```python
from build123d import *

# Parameters (mm, degrees)
SKETCH2_R                = 15.5
SKETCH2_R_2              = 14
BOSS_EXTRUDE1_DEPTH      = 25
SKETCH3_OUTSIDE_W        = 43.094
SKETCH3_OUTSIDE_H        = 43.094
CUT_EXTRUDE1_DEPTH       = 26
SKETCH5_R                = 2.5
CUT_EXTRUDE2_DEPTH       = 16.5
SKETCH6_R                = 2
BOSS_EXTRUDE2_DEPTH      = 1.5
BOSS_EXTRUDE2_DEPTH_BACK = 1.5
FILLET1_R                = 1


with BuildPart() as part:
    # Sketch2 → Boss-Extrude1 (new body)
    with BuildSketch(Plane(origin=(0, 0, 0), x_dir=(1, 0, 0), z_dir=(0, 1, 0))):
        Circle(SKETCH2_R)
        Circle(SKETCH2_R_2, mode=Mode.SUBTRACT)
    extrude(amount=BOSS_EXTRUDE1_DEPTH)

    # Sketch3 outside → Cut-Extrude1 (cut, through all)
    with BuildSketch(Plane(origin=(0, 25, 0), x_dir=(1, 0, 0), z_dir=(0, 1, 0))):
        Rectangle(SKETCH3_OUTSIDE_W, SKETCH3_OUTSIDE_H)
        with BuildLine():
            Line((0, 0), (7.5, 13.564659966))
            ThreePointArc((7.5, 13.564659966), (0, 15.5), (-7.5, 13.564659966))
            Line((-7.5, 13.564659966), (0, 0))
        make_face(mode=Mode.SUBTRACT)
    extrude(amount=-CUT_EXTRUDE1_DEPTH, mode=Mode.SUBTRACT)

    # Sketch5 → Cut-Extrude2 (cut, through all)
    with BuildSketch(Plane.XY):
        with Locations((0, 20)):
            Circle(SKETCH5_R)
        with Locations((0, 5)):
            Circle(SKETCH5_R)
    extrude(amount=-CUT_EXTRUDE2_DEPTH, mode=Mode.SUBTRACT)

    # Sketch6 → Boss-Extrude2 (add, two sides)
    with BuildSketch(Plane(origin=(0, 7.5, 0), x_dir=(0, 1, 0), z_dir=(-1, 0, 0))) as boss_extrude2_sk:
        with BuildLine():
            Line((2, 20.5), (2, 15.25))
            Line((2, 15.25), (8, 15.25))
            Line((8, 15.25), (8, 20.5))
            ThreePointArc((8, 20.5), (5, 23.5), (2, 20.5))
        make_face()
        with Locations((5, 20.5)):
            Circle(SKETCH6_R, mode=Mode.SUBTRACT)
    extrude(amount=BOSS_EXTRUDE2_DEPTH)
    extrude(boss_extrude2_sk.sketch, amount=-BOSS_EXTRUDE2_DEPTH_BACK)

    # Fillet1
    fillet1_edges = [part.edges().sort_by_distance(p)[0] for p in [
        (-1.5, 12.5, -15.427248621),
        (1.5, 12.5, -15.427248621),
    ]]
    fillet(fillet1_edges, radius=FILLET1_R)


solid = part.part
```
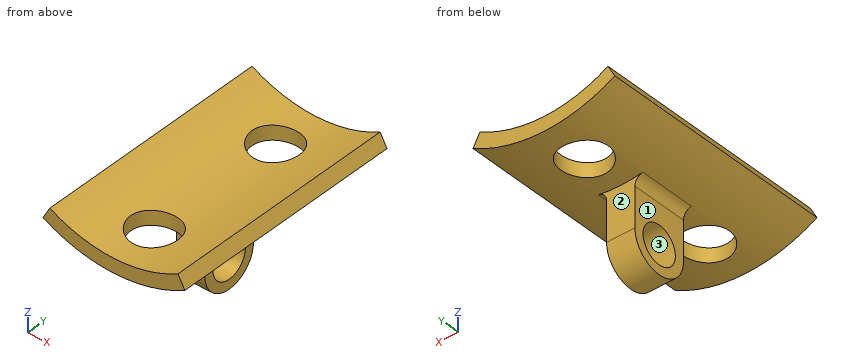
Part model, mm, in its own coordinate system. Face numbers are marked on the shaded views. Round coordinates to 2 decimals unless told otherwise and drop trailing zeros. Write each loop counter-clockwise with the first axis right and the second up, starting at its lowest first coordinate (ties: lowest second). Pieces come first, ordered by that corner, then holes. Notation, with made-up numbers: (52, -33) -> (71, -33) arc R9 cw to (71, -25) -> close; hole circle Ø6 at (18, -28). An arc over 180 degrees is marked (long way). Return JSON: item names as keys, results as strings. Group by question number.
Q1. Pin check, flat tips, straight feed: pin 1 (4 mm diameter, centred on x = 1.5, z = -18, fed in from -Y); pin 2 (1.5 mm diameter, centred on y = 12.5, z = -17.5, fed in from +X); pin 3 (6.5 mm diameter, centred on x = 0, y = 20, fed in from +Z). Stop position of each tip, or through.
Q2. Saw through at A-A on x = 0. Write the cut outline in (y, z), plus the area to 3 significant figures.
Q3. Saw through at B-B on y = 12.5. Write the cut outline in (x, z), plus the area to 3 significant figures.
Q4. Probe L1, parallel to Y at x = -0.25, z = -20.5; L2, parallel to Z at x = -0.2, y = 12.5; L3, parallel to Z at x = -1.25, y = 14. List the from-to ranges inside material, lowest first. Write a range as [from, to].
Q5. Mould opens along Y. For the marked faces 1, 2 and 3 say: pulls with the +Y half, pulls with the -Y half, needs draft (parallel to the pull), parting line crosses it, or undercut.
Q6. Saw through at D-D on x = 2. Write the cut outline in (y, z), plus the area to 3 significant figures.
Q7. Saw through at C-C on z = -21.75. Write the cut outline in (x, y).
Answer:
{
 "1": {"pin 1": "y = 9.5", "pin 2": "x = 1.5", "pin 3": "z = -13.62"},
 "2": {"outline": "(0, -15.5) -> (2.5, -15.5) -> (2.5, -14) -> (0, -14) -> close; (7.5, -15.5) -> (9.5, -15.5) -> (9.5, -20.5) arc R3 ccw to (15.5, -20.5) -> (15.5, -15.5) -> (17.5, -15.5) -> (17.5, -14) -> (7.5, -14) -> close; (22.5, -15.5) -> (25, -15.5) -> (25, -14) -> (22.5, -14) -> close; hole circle Ø4 at (12.5, -20.5)", "area": "54.1 mm2"},
 "3": {"outline": "(-7.5, -13.56) arc R15.5 ccw to (-2.35, -15.32) arc R1 cw to (-1.5, -16.31) -> (-1.5, -18.5) -> (1.5, -18.5) -> (1.5, -16.31) arc R1 cw to (2.35, -15.32) arc R15.5 ccw to (7.5, -13.56) -> (6.77, -12.25) arc R14 cw to (-6.77, -12.25) -> close; (-1.5, -23.5) -> (1.5, -23.5) -> (1.5, -22.5) -> (-1.5, -22.5) -> close", "area": "34.7 mm2"},
 "4": {"L1": "[9.5, 10.5], [14.5, 15.5]", "L2": "[-23.5, -22.5], [-18.5, -14]", "L3": "[-23.1, -21.82], [-19.18, -13.94]"},
 "5": {"face 1": "needs draft", "face 2": "pulls with the +Y half", "face 3": "undercut"},
 "6": {"outline": "(0, -15.37) -> (3.5, -15.37) -> (3.5, -13.86) -> (0, -13.86) -> close; (6.5, -15.37) -> (9.5, -15.37) -> (9.5, -15.44) -> (15.5, -15.44) -> (15.5, -15.37) -> (18.5, -15.37) -> (18.5, -13.86) -> (6.5, -13.86) -> close; (21.5, -15.37) -> (25, -15.37) -> (25, -13.86) -> (21.5, -13.86) -> close", "area": "29.2 mm2"},
 "7": {"outline": "(-1.5, 9.77) -> (1.5, 9.77) -> (1.5, 10.94) -> (-1.5, 10.94) -> close; (-1.5, 14.06) -> (1.5, 14.06) -> (1.5, 15.23) -> (-1.5, 15.23) -> close"}
}
